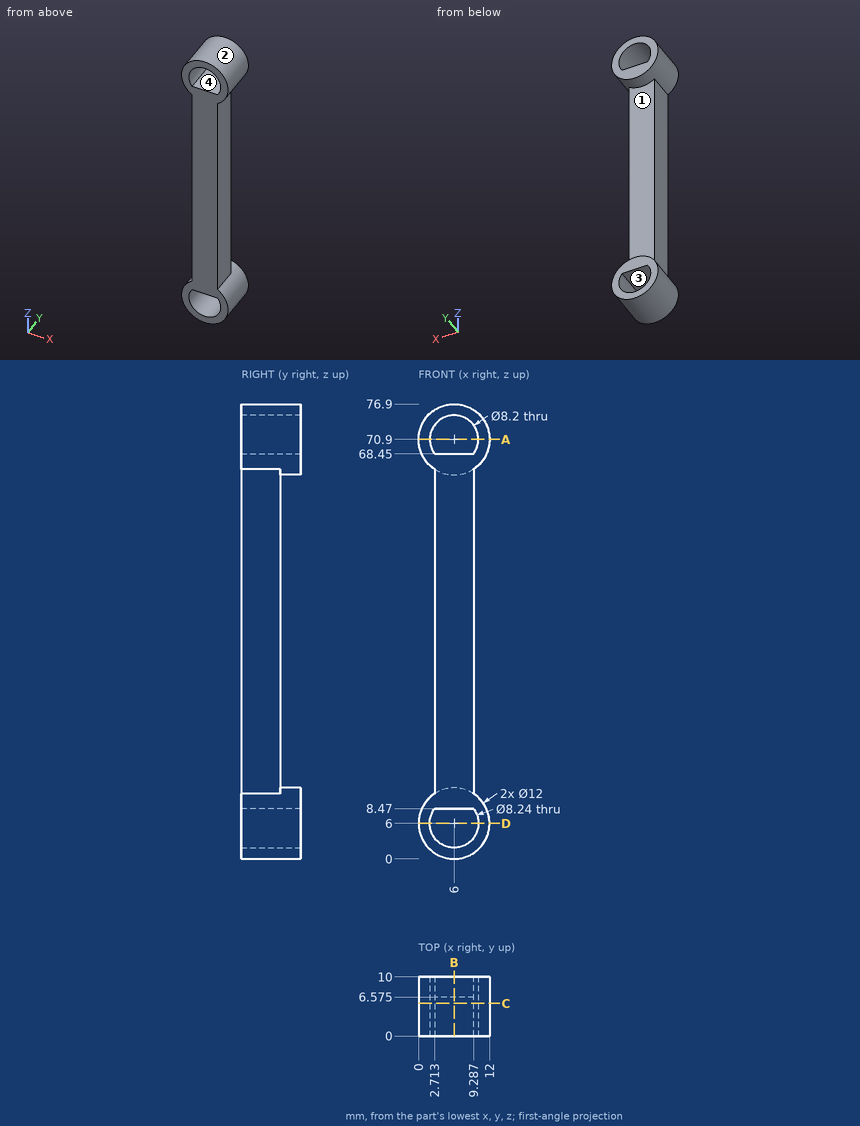
Verification items for this drawing (mm, ordinates from the low corner). Coordinates: 2 decimals unless noted, no trailing zeros. Write each loop counter-clockwise with the first axis right and the second up, starting at its lowest first coordinate (ties: lowest second). Pieces come first, ordered by that corner, then holes. Notation, with made-up numbers: (-20.5, -9) -> (31.5, -9) arc R23 ccw to (31.5, 11) -> close; hole circle Ø9 at (86, -9.5). An arc over 180 degrees is marked (long way). One line per item, written item: value. Start each with the question number.
Q1. Go/stop test with flat-tipped pins: P1, Ø3, axis at x = 2, y = 6.5, coming from the +Z side (1 decimal); P2, Ø4, axis at x = 3, y = 3.5, coming from the -Z side; P3, Ø1, axis at y = 5, z = 9.5, coming from the -X side (1 decimal). Record where each tip stops, or that it passes through.
Q2. Cross-section at A-A on z = 70.9. Enter the section's corners in (x, y).
Q3. Cross-section at B-B on x = 6. State how many separate pieces and enclosed holes the cut face has.
Q4. Mould release check, pull along X, two halves, no side actions. Record for the marked faces 1, 2, 3 and 4: pulls with the +X half, pulls with the -X half, needs draft (parallel to the pull), parting line crosses it, or undercut.
Q5. Cross-section at D-D on z = 6. Enter the section's corners in (x, y), and give its area (3 significant figures).
Q6. Thickness scan on L1, parallel to X at y = 7.75, z = 6; L2, parallel to Z at x = 9.5, y = 8.25 (1 decimal); L3, parallel to Z at x = 5.5, y = 7.5. Record the ranges inside material, lowest first. Write a range as from..to.
Q7. Cross-section at C-C on y = 5.5. Enter the section's corners in (x, z).
Checked values:
1. P1: stops at z = 76.4
1. P2: stops at z = 0.08
1. P3: stops at x = 0.8
2. outline: (0, 0) -> (1.9, 0) -> (1.9, 10) -> (0, 10) -> close; (10.1, 0) -> (12, 0) -> (12, 10) -> (10.1, 10) -> close
3. separate pieces: 3
3. enclosed holes: 0
4. face 1: needs draft
4. face 2: parting line crosses it
4. face 3: undercut
4. face 4: undercut
5. outline: (0, 0) -> (1.88, 0) -> (1.88, 10) -> (0, 10) -> close; (10.12, 0) -> (12, 0) -> (12, 10) -> (10.12, 10) -> close
5. area: 37.6 mm²
6. L1: x = 0..1.88, 10.12..12
6. L2: z = 1.1..3.8, 8.2..10.9, 66..68.8, 73..75.8
6. L3: z = 0.02..1.91, 8.47..11.98, 64.92..68.45, 74.97..76.88
7. outline: (2.71, 11.02) arc R6 ccw (long way) to (9.29, 11.02) -> (9.29, 65.88) arc R6 ccw (long way) to (2.71, 65.88) -> close; hole (2.7, 8.47) arc R4.12 ccw (long way) to (9.3, 8.47) -> close; hole (2.71, 68.45) -> (9.29, 68.45) arc R4.1 ccw (long way) to start
